CAD build for the part. Positions are in the model's coordinates, mm. A direction names the side the tool comes from. Give positions to 0.01 mm unless a question says otherwise; leave off trailing zeros. Order: outer loops, then holes, each group sorted by start corner. A loop starts at its lowest first (then second) coordinate and runs counter-clockwise, first axis right, second up.
```python
from build123d import *

# Parameters (mm, degrees)
SKETCH1_R                     = 10
BOSS_EXTRUDE1_DEPTH           = 26
BOSS_EXTRUDE1_TAPER           = 1
BOSS_EXTRUDE1_OTHER_WAY_DEPTH = 6
BOSS_EXTRUDE1_OTHER_WAY_TAPER = -1
CUT_EXTRUDE1_DEPTH            = 30.668352709
CUT_EXTRUDE1_DEPTH_BACK       = 30.668352709
SKETCH3_W                     = 10
SKETCH3_H                     = 6
CUT_EXTRUDE2_DEPTH            = 25
CUT_EXTRUDE3_DEPTH            = 32.721577304
CUT_EXTRUDE3_DEPTH_BACK       = 32.721577304
SKETCH4_R                     = 1.5
FILLET2_SIZE                  = 5
CUT_EXTRUDE5_DEPTH            = 30.668352865
CUT_EXTRUDE5_DEPTH_BACK       = 30.668352865
SKETCH8_W                     = 10
SKETCH8_H                     = 6
CUT_EXTRUDE6_DEPTH            = 30.976934008
CUT_EXTRUDE7_DEPTH            = 30.632846395
CUT_EXTRUDE8_DEPTH            = 32.688371532
CUT_EXTRUDE8_DEPTH_BACK       = 32.688371532
SKETCH9_R                     = 1.351518808
FILLET3_SIZE                  = 5
SKETCH10_R                    = 1
CUT_EXTRUDE9_DEPTH            = 30.623606957


with BuildPart() as part:
    # Sketch1 → Boss-Extrude1 (new body)
    with BuildSketch(Plane(origin=(0, 0, 0), x_dir=(1, 0, 0), z_dir=(0, 1, 0))):
        Circle(SKETCH1_R)
    extrude(amount=BOSS_EXTRUDE1_DEPTH, taper=BOSS_EXTRUDE1_TAPER)

    # Sketch1 → Boss-Extrude1 other way (add)
    with BuildSketch(Plane(origin=(0, 0, 0), x_dir=(1, 0, 0), z_dir=(0, 1, 0))):
        Circle(SKETCH1_R)
    extrude(amount=-BOSS_EXTRUDE1_OTHER_WAY_DEPTH, taper=BOSS_EXTRUDE1_OTHER_WAY_TAPER)

    # Sketch2 → Cut-Extrude1 (cut, two sides: drawn at the far end of the back side and taken through both)
    with BuildSketch(Plane(origin=(0, 0, 0), x_dir=(0, 0, -1), z_dir=(1, 0, 0)).offset(-CUT_EXTRUDE1_DEPTH_BACK)):
        Polygon((-0.453831688, 26), (-0.453831688, 20), (-13.188542788, 7.2652889), (-13.188542788, 26), align=None)
    extrude(amount=CUT_EXTRUDE1_DEPTH + CUT_EXTRUDE1_DEPTH_BACK, mode=Mode.SUBTRACT)

    # Sketch3 → Cut-Extrude2 (cut)
    with BuildSketch(Plane.XY.offset(0.453831688)):
        with Locations((0, 23)):
            Rectangle(SKETCH3_W, SKETCH3_H)
    extrude(amount=-CUT_EXTRUDE2_DEPTH, mode=Mode.SUBTRACT)

    # Sketch4 → Cut-Extrude3 (cut, two sides: drawn at the far end of the back side and taken through both)
    with BuildSketch(Plane(origin=(-5, 0, 0), x_dir=(0, 0, -1), z_dir=(1, 0, 0)).offset(-CUT_EXTRUDE3_DEPTH_BACK)):
        with Locations((2.046168312, 23.5)):
            Circle(SKETCH4_R)
    extrude(amount=CUT_EXTRUDE3_DEPTH + CUT_EXTRUDE3_DEPTH_BACK, mode=Mode.SUBTRACT)

    # Fillet2
    # a fillet whose section is not a circle: 5 mm, written as the material it takes off along each edge
    with BuildSketch(Plane(origin=(-7.5, 26, 0.453831688), x_dir=(0, -1, 0), z_dir=(1, 0, 0))) as fillet2_piece_1:
        with BuildLine():
            Bezier((FILLET2_SIZE, 0), (0, 0), (0, FILLET2_SIZE), weights=[1, 1.5, 1])
            Line((0, FILLET2_SIZE), (0, 0))
            Line((0, 0), (FILLET2_SIZE, 0))
        make_face()
    extrude(amount=29.535374468, mode=Mode.SUBTRACT)
    with BuildSketch(Plane(origin=(-22.035374468, 26, 0.453831688), x_dir=(0, 0, -1), z_dir=(1, 0, 0))) as fillet2_piece_2:
        with BuildLine():
            Bezier((FILLET2_SIZE, 0), (0, 0), (0, -FILLET2_SIZE), weights=[1, 1.5, 1])
            Line((0, -FILLET2_SIZE), (0, 0))
            Line((0, 0), (FILLET2_SIZE, 0))
        make_face()
    extrude(amount=29.535374468, mode=Mode.SUBTRACT)

    # Sketch7 → Cut-Extrude5 (cut, two sides: drawn at the far end of the back side and taken through both)
    with BuildSketch(Plane(origin=(0, 0, 0), x_dir=(0, 0, -1), z_dir=(1, 0, 0)).offset(-CUT_EXTRUDE5_DEPTH_BACK)):
        Polygon((-0.873019237, -6), (-0.873019237, 0), (-11.31781305, 10.444793812), (-11.31781305, -6), align=None)
    extrude(amount=CUT_EXTRUDE5_DEPTH + CUT_EXTRUDE5_DEPTH_BACK, mode=Mode.SUBTRACT)

    # Sketch8 → Cut-Extrude6 (cut, through all)
    with BuildSketch(Plane.XY.offset(0.873019237)):
        with Locations((0, -3)):
            Rectangle(SKETCH8_W, SKETCH8_H)
    extrude(amount=-CUT_EXTRUDE6_DEPTH, mode=Mode.SUBTRACT)

    # Sketch6 → Cut-Extrude7 (cut, through all)
    with BuildSketch(Plane(origin=(0, 20, 0), x_dir=(1, 0, 0), z_dir=(0, 1, 0))):
        with BuildLine():
            Line((5, 5.791049209), (5, -0.453831688))
            Line((5, -0.453831688), (-5, -0.453831688))
            Line((-5, -0.453831688), (-5, 5.791049209))
            ThreePointArc((-5, 5.791049209), (0, 7.650898701), (5, 5.791049209))
        make_face()
    extrude(amount=-CUT_EXTRUDE7_DEPTH, mode=Mode.SUBTRACT)

    # Sketch9 → Cut-Extrude8 (cut, two sides: drawn at the far end of the back side and taken through both)
    with BuildSketch(Plane(origin=(-5, 0, 0), x_dir=(0, 0, -1), z_dir=(1, 0, 0)).offset(-CUT_EXTRUDE8_DEPTH_BACK)):
        with Locations((1.626980763, -3.5)):
            Circle(SKETCH9_R)
    extrude(amount=CUT_EXTRUDE8_DEPTH + CUT_EXTRUDE8_DEPTH_BACK, mode=Mode.SUBTRACT)

    # Fillet3
    # a fillet whose section is not a circle: 5 mm, written as the material it takes off along each edge
    with BuildSketch(Plane(origin=(22.566946591, -6, 0.873019237), x_dir=(0, 0, -1), z_dir=(-1, 0, 0))) as fillet3_piece_1:
        with BuildLine():
            Bezier((FILLET3_SIZE, 0), (0, 0), (0, -FILLET3_SIZE), weights=[1, 1, 1])
            Line((0, -FILLET3_SIZE), (0, 0))
            Line((0, 0), (FILLET3_SIZE, 0))
        make_face()
    extrude(amount=30.066946591, mode=Mode.SUBTRACT)
    with BuildSketch(Plane(origin=(7.5, -6, 0.873019237), x_dir=(0, 1, 0), z_dir=(-1, 0, 0))) as fillet3_piece_2:
        with BuildLine():
            Bezier((FILLET3_SIZE, 0), (0, 0), (0, FILLET3_SIZE), weights=[1, 1, 1])
            Line((0, FILLET3_SIZE), (0, 0))
            Line((0, 0), (FILLET3_SIZE, 0))
        make_face()
    extrude(amount=30.066946591, mode=Mode.SUBTRACT)

    # Sketch10 → Cut-Extrude9 (cut, through all)
    with BuildSketch(Plane(origin=(0, 20, 0), x_dir=(1, 0, 0), z_dir=(0, 1, 0))):
        with Locations(Location((0, -2.56777392, 0), (0, 0, 270))):
            Circle(SKETCH10_R)
    extrude(amount=-CUT_EXTRUDE9_DEPTH, mode=Mode.SUBTRACT)


solid = part.part
```
Item 1: Two-plate mould, pull along Y, no slides. Class faces 4 (the face through (0, 20, -8)), 5 (the face through (7.257, 23.566, -0.548)), 6 (the face through (7.3, 20.5, 0.454)): released by +Y, released by -Y, zero draft, split by the parting line, or undercut.
Item 2: Slice it at B-B (x = 0). State how many separate pieces and enclosed holes the cut face has, and give its area (3 significant figures).
Item 3: Drop flat-ended pins along their axis: pin 1 Ø3.5 at (x, z) = (1.5, -8) entering from -Y; pin 2 Ø10 at (x, z) = (-2.5, -3.5) entering from +Y; pin 3 Ø5 at (y, z) = (5, -0.5) entering from +X; pin 4 Ø10 at (x, y) = (1.5, 20) entering from -Z. Give the stop position or say it passes through.
Item 4: Slice it at A-A (y = 6). Give the cut face in (x, z), and give its area (3 significant figures).
Item 5: Tool access for faces 1 (the face through (-1.28, 9.776, -9.746)), 2 (the face through (-7.4, 20.5, 0.454)), 3 (the face through (7.5, -0.5, 0.873)): list every direction of +Z, -Z, +X, -X, +Y, -Y with a clear straight run to the whole face (end or side of a thin tool).
Item 6: Wall check: L1, parallel to Z at x = 0, y = 13.25; L2, parallel to Y at x = -5.75, z = -1.25; L3, parallel to Z at x = 7.7, y = 23.5. Give the ranges that are in metal, low to high.
A:
1. face 4: released by +Y
1. face 5: undercut
1. face 6: zero draft
2. separate pieces: 3
2. enclosed holes: 0
2. area: 115 mm2
3. pin 1: stops at y = 0
3. pin 2: stops at y = 26
3. pin 3: stops at x = 9.96
3. pin 4: stops at z = -9.73
4. outline: (-7.12, 6.87) arc R9.9 ccw (long way) to (7.12, 6.87) - close; hole (-5, -5.79) arc R7.65 ccw to (5, -5.79) - (5, 0.45) - (-5, 0.45) - close; hole circle Ø2 at (0, 2.57)
4. area: 200 mm2
5. face 1: +Y
5. face 2: +Z, +X, -X, +Y
5. face 3: +Z, +X, -X, -Y
6. L1: z = -9.77 to -7.65, 0.45 to 1.57, 3.57 to 7.2
6. L2: y = -5.39 to -4.8, -2.2 to 22.23, 24.77 to 25.49
6. L3: z = -5.72 to -3.55, -0.55 to 0.22
